Geometry check sheet. Reference: drawing and pictorial views, mm from the part's lowest x, y, z. A direction names the side the tool comes from. Give positions to 0.01 mm unless a question says otherwise; leave off trailing zeros. Write each loop counter-clockwise with the first axis right and the second up, starting at its lowest first coordinate (ties: lowest second). Pieces come first, ordered by that corner, then holes. Notation, with made-up numbers: (53, 83) -> (92, 83) arc R19 cw to (92, 87) -> close; hole circle Ø8 at (44.25, -15). An arc over 180 degrees is marked (long way). Write each question's results on one line, items separated by ' | '. Start each with the question number.
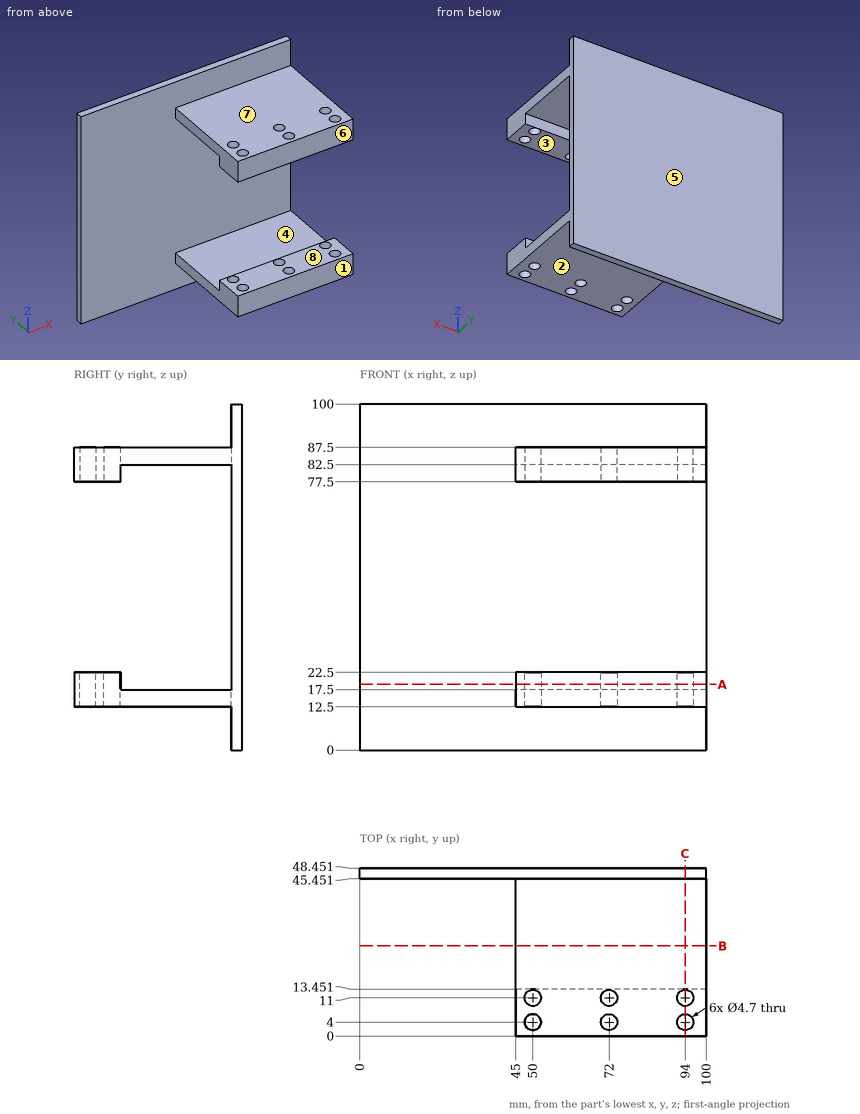
Item 1: Section check B-B on y = 26. Record the boundary of the cut face in (x, z), then the cut area to 3 significant figures.
Item 2: Set-up check for the marked faces 4, 5, 6, 7 and 8: record each of +Z, -Z, +X, -X, +Y, -Y from which the full face is reachable in a straight line by a thin tool's end or side.
Item 3: Thickness scan on probe 1 along Y at (x, z) = (50, 83.75); probe 2 along Z at (x, y) = (72, 40); probe 3 along Z at (x, y) = (81, 5.5). Record the ranges inside material, lowest first. Write a range as from..to.
Item 4: Mould release check, pull along Z, two halves, no side actions. Record for the marked faces 1, 2 and 3: pulls with the +Z half, pulls with the -Z half, needs draft (parallel to the pull), parting line crosses it, or undercut.
Item 5: Section check A-A on z = 19. Record the boundary of the cut face in (x, y).
Item 6: Depth check by flat-ended pin: pin 1 Ø15 at (x, y) = (74.5, 6.5) entering from +Z; pin 2 Ø15 at (x, y) = (67.5, 4) entering from -Z; pin 3 Ø5 at (x, z) = (63, 39.5) entering from -Y. Enter the tip coordinate at first touch or a pass-through.
Item 7: Section check C-C on x = 94. Count the separate pieces of the cut face and the enclosed holes in it, then the cut area to 3 significant figures.
Check sheet entries:
1) outline: (45, 12.5) -> (100, 12.5) -> (100, 17.5) -> (45, 17.5) -> close; (45, 82.5) -> (100, 82.5) -> (100, 87.5) -> (45, 87.5) -> close | area: 550 mm^2
2) face 4: +X, -X | face 5: +Z, -Z, +X, -X, +Y | face 6: +Z, -Z, +X, -X, -Y | face 7: +Z, +X, -X, -Y | face 8: +X, -X, -Y
3) probe 1: y = 0..1.65, 6.35..8.65, 13.35..48.45 | probe 2: z = 12.5..17.5, 82.5..87.5 | probe 3: z = 12.5..22.5, 77.5..87.5
4) face 1: needs draft | face 2: pulls with the -Z half | face 3: undercut
5) outline: (0, 45.45) -> (100, 45.45) -> (100, 48.45) -> (0, 48.45) -> close; (45, 0) -> (100, 0) -> (100, 13.45) -> (45, 13.45) -> close; hole circle Ø4.7 at (50, 4); hole circle Ø4.7 at (50, 11); hole circle Ø4.7 at (72, 4); hole circle Ø4.7 at (72, 11); hole circle Ø4.7 at (94, 4); hole circle Ø4.7 at (94, 11)
6) pin 1: stops at z = 87.5 | pin 2: stops at z = 12.5 | pin 3: stops at y = 45.45
7) separate pieces: 5 | enclosed holes: 0 | area: 701 mm^2
